Check sheet for the modelled part. Datum: model origin and axes. Units: mm. Give positions to 0.01 mm unless a question says otherwise; leave off trailing zeros. Loops run counter-clockwise (first coordinate to the right, second up) from the corner with the lowest first, then second, coordinate; pieces in that order, holes last. Notation, with made-up numbers: (78, -33.75) -> (126, -33.75) arc R16 ccw to (126, -7.75) -> close; hole circle Ø8 at (49.5, -10.5). An arc over 180 degrees is marked (long way). Write each question's results on one line, items separated by ' | '. Start each with the question number.
Item 1: Gauge pin test, flat ends, axial feed: pin 1 Ø0.6 at (x, z) = (6.35, 21.75) entering from -Y; pin 2 Ø1.5 at (x, z) = (0, 6) entering from -Y; pin 3 Ø0.9 at (x, y) = (-3, 2) entering from -Z. Record the tip position at first contact, or that the pin passes through.
Item 2: Scan lines: line 1 along Z through (x, y) = (-12.5, 0.45); line 2 along Z through (x, y) = (5.75, 1.55); line 3 along X through (y, z) = (-0.5, -12.5). Record each from-to range of solid material in increasing order.
Item 3: Cross-section at B-B on z = 20.75. Enter the section's corners in (x, y), then the cut area to 3 significant figures.
Item 4: Cross-section at A-A on y = 0.65. State how many separate pieces and enclosed holes the cut face has, then the cut area to 3 significant figures.
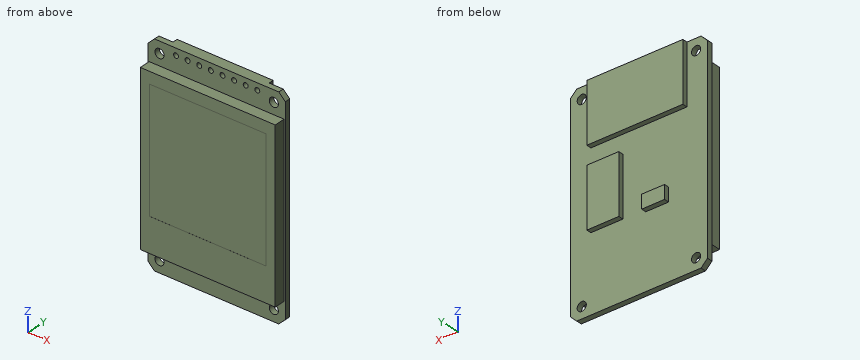
Solid Edge part; units mm, degrees
sketch "Sketch1" plane through (0, 0, 0) normal (0, -1, 0) x (1, 0, 0)
  line L0 (-13.59, -23.25) -> (-15, -21.84)
  line L1 (-15, 21.84) -> (-15, -21.84)
  line L2 (-15, 21.84) -> (-13.59, 23.25)
  line L3 (13.59, 23.25) -> (-13.59, 23.25)
  line L4 (13.59, 23.25) -> (15, 21.84)
  line L5 (15, -21.84) -> (15, 21.84)
  line L6 (13.59, -23.25) -> (15, -21.84)
  line L7 (-13.59, -23.25) -> (13.59, -23.25)
extrude "Protrusion1" add sketch "Sketch1" against normal blind 1.2
sketch "Sketch2" plane through (0, 0, 0) normal (0, -1, 0) x (1, 0, 0)
  line L0 (14.75, 18.25) -> (-14.75, 18.25)
  line L1 (-14.75, 18.25) -> (-14.75, -18.25)
  line L2 (-14.75, -18.25) -> (14.75, -18.25)
  line L3 (14.75, -18.25) -> (14.75, 18.25)
extrude "ExtrudedProtrusion_2" add sketch "Sketch2" along normal blind 2.4
sketch "Sketch3" plane through (0, 0, 0) normal (0, -1, 0) x (1, 0, 0)
  circle A0 centre (-12.5, 20.75) radius 1
  circle A1 centre (12.5, 20.75) radius 1
  circle A2 centre (12.5, -20.75) radius 1
  circle A3 centre (-12.5, -20.75) radius 1
extrude "Cutout1" cut sketch "Sketch3" against normal up to next
sketch "Sketch4" plane through (0, -2.4, 0) normal (0, -1, 0) x (1, 0, 0)
  line L0 (12.75, 15.69) -> (-12.75, 15.69)
  line L1 (-12.75, 15.69) -> (-12.75, -10.81)
  line L2 (-12.75, -10.81) -> (12.75, -10.81)
  line L3 (12.75, -10.81) -> (12.75, 15.69)
extrude "ExtrudedCutout_2" cut sketch "Sketch4" against normal blind 0.01
sketch "Sketch5" plane through (0, 0, 0) normal (0, -1, 0) x (1, 0, 0)
  circle A0 centre (-8.89, 21.75) radius 0.5381
  circle A1 centre (-6.35, 21.75) radius 0.5381
  circle A2 centre (-3.81, 21.75) radius 0.5381
  circle A3 centre (-1.27, 21.75) radius 0.5381
  circle A4 centre (1.27, 21.75) radius 0.5381
  circle A5 centre (3.81, 21.75) radius 0.5381
  circle A6 centre (6.35, 21.75) radius 0.5381
  circle A7 centre (8.89, 21.75) radius 0.5381
extrude "Cutout2" cut sketch "Sketch5" against normal through all
sketch "Sketch6" plane through (0, 1.2, 0) normal (0, 1, 0) x (0, 0, 1)
  line L0 (10.25, -10.5) -> (10.25, 10.5)
  line L1 (10.25, 10.5) -> (23.25, 10.5)
  line L2 (23.25, 10.5) -> (23.25, 7.6087)
  line L3 (23.25, 7.6087) -> (23.25, -7.6326)
  line L4 (23.25, -7.6326) -> (23.25, -10.5)
  line L5 (23.25, -10.5) -> (10.25, -10.5)
  line L6 (-6.75, 3.5) -> (6.25, 3.5)
  line L7 (6.25, 3.5) -> (6.25, 10.5)
  line L8 (6.25, 10.5) -> (-6.75, 10.5)
  line L9 (-6.75, 10.5) -> (-6.75, 3.5)
  line L10 (-7.25, -1.5) -> (-4.25, -1.5)
  line L11 (-4.25, -1.5) -> (-4.25, -6.5)
  line L12 (-4.25, -6.5) -> (-7.25, -6.5)
  line L13 (-7.25, -6.5) -> (-7.25, -1.5)
extrude "ExtrudedProtrusion_6" add sketch "Sketch6" along normal blind 1.1
properties material "Polycarbonate"
Answer sheet:
1) pin 1: stops at y = 1.2 | pin 2: stops at y = -2.39 | pin 3: stops at z = -7.25
2) line 1: z = -23.25 to -21.75, -19.75 to 19.75, 21.75 to 23.25 | line 2: z = -6.75 to 6.25, 10.25 to 23.25 | line 3: x = -14.75 to 14.75
3) outline: (-15, 0) -> (-13.5, 0) -> (-13.5, 1.2) -> (-15, 1.2) -> close; (-11.5, 0) -> (11.5, 0) -> (11.5, 1.2) -> (10.5, 1.2) -> (10.5, 2.3) -> (-10.5, 2.3) -> (-10.5, 1.2) -> (-11.5, 1.2) -> close; (13.5, 0) -> (15, 0) -> (15, 1.2) -> (13.5, 1.2) -> close | area: 54.3 mm²
4) separate pieces: 1 | enclosed holes: 12 | area: 1,370 mm²
